The model under review builds one solid part; all positions refer to its coordinate system, in mm. Face numbers are marked on the shaded views. A direction names the side the tool comes from. Round coordinates to 2 decimals unless told otherwise and drop trailing zeros. Loops run counter-clockwise (first coordinate to the right, second up) from the corner with the lowest first, then second, coordinate; pieces in that order, holes last. Notation, with made-up numbers: (86.25, 0) - (140.25, 0) arc R23 cw to (140.25, 10) - close; hole circle Ø10 at (24.5, 74). An arc over 180 degrees is marked (long way). Answer as CSV lines item,"result".
Autodesk Inventor part; units mm, degrees
ref_plane "YZ Plane" through (0, 0, 0) normal (1, 0, 0) x (0, 1, 0)
ref_plane "XZ Plane" through (0, 0, 0) normal (0, 1, 0) x (-1, 0, 0)
ref_plane "XY Plane" through (0, 0, 0) normal (0, 0, 1) x (1, 0, 0)
sketch "Sketch1" plane through (0, 0, 0) normal (0, 0, 1) x (1, 0, 0)
  line L0 (-17.9641, 33.2251) -> (-14.7891, 33.2251)
  line L1 (-14.7891, 33.2251) -> (-14.7891, -17.5749)
  line L2 (-14.7891, -17.5749) -> (-17.9641, -17.5749)
  line L3 (-17.9641, -17.5749) -> (-17.9641, 33.2251)
  point P0 (0, 0)
  dimension "d0" = 3.175
  dimension "d1" = 50.8
revolve "Revolution1" add sketch "Sketch1" angle 360 about axis through (-17.9641, -17.5749, 0) along (0, 1, 0)
sketch "Sketch2" plane through (-17.9641, 33.2251, 0) normal (0, 1, 0) x (1, 0, 0)
  circle A0 centre (0, 0) radius 3.175
  line L0 (-2.7933, -6.7141) -> (-7.2112, -0.938)
  line L1 (-7.2112, -0.938) -> (-4.418, 5.7761)
  line L2 (-4.418, 5.7761) -> (2.7933, 6.7141)
  line L3 (2.7933, 6.7141) -> (7.2112, 0.938)
  line L4 (7.2112, 0.938) -> (4.418, -5.7761)
  line L5 (4.418, -5.7761) -> (-2.7933, -6.7141)
  point P0 (17.9641, 0)
extrude "Extrusion1" add sketch "Sketch2" along normal blind 3.81 contours A0 | L0 L1 L2 L3 L4 L5
thread "Thread1"
sketch "Sketch3" plane through (-17.9641, 37.0351, 0) normal (0, 1, 0) x (1, 0, 0)
  spline S0 degree 5 poles (-1.6705, -1.7697) (-1.5087, -1.85) (-0.562, -1.832) (2.4108, -1.3359) (-1.0538, -0.5942) (-0.3082, 0.5963) (2.0933, -0.7076) (-1.4851, 3.8244) (-2.0876, 1.526) (-0.2865, 2.0954) (0.0858, 0.4541) (-1.2327, 0.9989) (-1.1868, -0.5585) (0.1138, -0.9114) (-0.367, -1.1465) (-1.6028, -1.5407) (-1.7853, -1.7128) (-1.6705, -1.7697) knots 0 0 0 0 0 0 0.118263 0.184405 0.277398 0.35545 0.432093 0.511849 0.589546 0.655005 0.725096 0.791185 0.859928 0.916088 1 1 1 1 1 1
  point P0 (17.9641, 0)
  point P1 (-0.2467, -0.2687)
  point P2 (-0.1215, 0.0477)
  point P3 (0.7392, 0.3)
  point P4 (-1.3859, 2.4418)
  point P5 (-1.4827, 2.0902)
  point P6 (-0.4576, 1.5038)
  point P7 (-0.3161, 0.9046)
  point P8 (-0.8855, 0.5658)
  point P9 (-0.8855, -0.3278)
  point P10 (-0.3187, -0.9153)
  point P11 (-0.8855, -1.3006)
extrude "Extrusion2" cut sketch "Sketch3" against normal blind 0.254
properties part number ".25 diameter 2'' bolt"
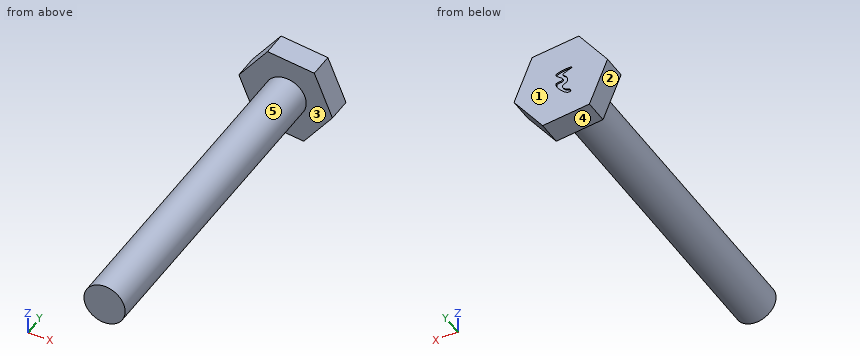
1. Clearance check with flat-ended pins moving along their axes: pin 1 (3 mm diameter, centred on y = 2, z = 3, fed in from +X); pin 2 (1.5 mm diameter, centred on x = -20, y = 8.5, fed in from -Z); pin 3 (4 mm diameter, centred on y = 27, z = 1, fed in from -X). State where each tip first meets the part, or that it passes through.
Numbers:
pin 1,"stops at x = -15.17"
pin 2,"stops at z = -2.9"
pin 3,"stops at x = -21.14"
2. Take a section at A-A (y = 25). State the section outline as (x, z) points (3 decimals).
Numbers:
outline,"circle Ø6.35 at (-17.964, 0)"
3. Take a section at B-B (z = -5.25). State the section outline as (x, y) points.
Numbers:
outline,"(-22.6, 33.23) - (-14.05, 33.23) - (-14.05, 37.04) - (-22.6, 37.04) - close"
4. Tool access review of the marked faces 4 and 5: name each direction out of +Z, -Z, +X, -X, +Y, -Y from which nothing blocks a thin tool from reaching the whole face with its end or side.
Numbers:
face 4,"-Z, -X, +Y, -Y"
face 5,"-Y"
5. Wall thickness on probe 1 along Y at (x, z) = (-18.25, 6.25); probe 2 along X at (y, z) = (8.5, 1.5); probe 3 along Z at (x, y) = (-16, -13.5): over which ranges is each line inside the solid? List them lowest first.
Numbers:
probe 1,"y = 33.23 to 37.04"
probe 2,"x = -20.76 to -15.17"
probe 3,"z = -2.49 to 2.49"
6. Draft analysis for pull direction Y (two halves, no side actions). For the marked faces 1, 2 and 3, state which applies: +Y half, -Y half, draft (parallel to the pull), parting line (faces both ways), or undercut.
Numbers:
face 1,"+Y half"
face 2,"draft"
face 3,"-Y half"
7. Take a section at C-C (z = 4.25). State the section outline as (x, y) points, plus the area to 3 significant figures.
Numbers:
outline,"(-22.64, 33.23) - (-12.91, 33.23) - (-12.91, 37.04) - (-22.64, 37.04) - close"
area,"37.1 mm²"
